Build history of the part. All positions in model axes, mm. A direction names the side the tool comes from. Round coordinates to 2 decimals unless told otherwise and drop trailing zeros. Loops run counter-clockwise (first coordinate to the right, second up) from the corner with the lowest first, then second, coordinate; pieces in that order, holes last. Notation, with made-up numbers: (71, 51.25) - (100, 51.25) arc R30 ccw to (100, 75.25) - close; hole circle Ø1 at (63.25, -33.75). An arc over 180 degrees is marked (long way). Use a Markdown table: item, result.
from build123d import *

# Parameters (mm, degrees)
F0_W          = 59.5
F0_H          = 29.5
F1_DEPTH      = 12.7
F1_DEPTH_BACK = 41.3
F2_R          = 3
F3_DEPTH      = 4.3
F4_R          = 1.5
F5_DEPTH      = 7.8


with BuildPart() as f1:
    # F0 (on Top) → F1 (new body, two sides)
    with BuildSketch(Plane.XY) as f1_sk:
        Rectangle(F0_W, F0_H)
    extrude(amount=F1_DEPTH)
    extrude(f1_sk.sketch, amount=-F1_DEPTH_BACK)

    # F2 (on Top) → F3 (join)
    with BuildSketch(Plane.XY):
        with BuildLine():
            Line((-35.5, -14.75), (35.5, -14.75))
            ThreePointArc((35.5, -14.75), (36.914214, -14.164214), (37.5, -12.75))
            Line((37.5, -12.75), (37.5, 12.75))
            ThreePointArc((37.5, 12.75), (36.914214, 14.164214), (35.5, 14.75))
            Line((35.5, 14.75), (-35.5, 14.75))
            ThreePointArc((-35.5, 14.75), (-36.914214, 14.164214), (-37.5, 12.75))
            Line((-37.5, 12.75), (-37.5, -12.75))
            ThreePointArc((-37.5, -12.75), (-36.914214, -14.164214), (-35.5, -14.75))
        make_face()
        with Locations((-33.476662, -8.75)):
            Circle(F2_R, mode=Mode.SUBTRACT)
        with Locations((34.023338, -8.75)):
            Circle(F2_R, mode=Mode.SUBTRACT)
        with Locations((-33.476662, 8.75)):
            Circle(F2_R, mode=Mode.SUBTRACT)
        with Locations((34.023338, 8.75)):
            Circle(F2_R, mode=Mode.SUBTRACT)
    extrude(amount=F3_DEPTH)

    # F4 (on face) → F5 (join)
    with BuildSketch(Plane.XY.offset(12.7)):
        with Locations((-16.25, 0)):
            Circle(F4_R)
    extrude(amount=F5_DEPTH)


solid = f1.part
Q1. Probe line 1 (Y direction, x = 32, z = 1.5); line 2 (Z direction, x = -13, y = 13); line 3 (X direction, y = -5, z = -12.5). List the from-to ranges inside material, lowest first.
Results found:
| item | result |
|---|---|
| line 1 | y = -14.75 to -10.96, -6.54 to 6.54, 10.96 to 14.75 |
| line 2 | z = -41.3 to 12.7 |
| line 3 | x = -29.75 to 29.75 |
Q2. Pull direction Y, two halves, no side cores. Call faces 5 (the face through (31.026, -8.618, 2.12)), 6 (the face through (0, 0, 12.7)), 7 (the face through (36.93, 14.15, 2.12)), 8 (the face through (-36.474, 8.882, 2.12)): pulls with the +Y half, pulls with the -Y half, needs draft (parallel to the pull), parting line crosses it, or undercut.
Results found:
| item | result |
|---|---|
| face 5 | undercut |
| face 6 | needs draft |
| face 7 | pulls with the +Y half |
| face 8 | undercut |
Q3. Which spindle directions (+Z, -Z, +X, -X, +Y, -Y) get a long thin tool onto all of the face, cutting with end or side? Do faces 1 (the face through (34, 0, 4.3)), 2 (the face through (-29.75, 0, -20)), 3 (the face through (-17.75, 0.07, 16.55)), 4 (the face through (34, 0, 0)). Say none if no direction does.
Results found:
| item | result |
|---|---|
| face 1 | +Z, +X, +Y, -Y |
| face 2 | -Z, -X, +Y, -Y |
| face 3 | +Z |
| face 4 | -Z, +X, +Y, -Y |
Q4. Cut at B-B, the plane x = -16.25. List the corners of the cut face in (y, z).
Results found:
| item | result |
|---|---|
| outline | (-14.75, -41.3) - (14.75, -41.3) - (14.75, 12.7) - (1.5, 12.7) - (1.5, 20.5) - (-1.5, 20.5) - (-1.5, 12.7) - (-14.75, 12.7) - close |
Q5. Drop flat-ended pins along their axis: pin 1 (3 mm diameter, centred on x = 17.5, y = -11, fed in from +Z); pin 2 (4 mm diameter, centred on x = 34.5, y = -7, fed in from +Z); pin 3 (2.5 mm diameter, centred on y = -2, z = 8, fed in from -X); pin 4 (3.5 mm diameter, centred on x = 34.02, y = 8.75, fed in from -Z). Give the stop position or say it passes through.
Results found:
| item | result |
|---|---|
| pin 1 | stops at z = 12.7 |
| pin 2 | stops at z = 4.3 |
| pin 3 | stops at x = -29.75 |
| pin 4 | passes through |
Q6. Cut at D-D, the plane z = -16. List the corners of the cut face in (x, y), plus the area to 3 significant figures.
Results found:
| item | result |
|---|---|
| outline | (-29.75, -14.75) - (29.75, -14.75) - (29.75, 14.75) - (-29.75, 14.75) - close |
| area | 1,760 mm2 |
Q7. Cut at A-A, the plane y = 8.75. List the corners of the cut face in (x, z).
Results found:
| item | result |
|---|---|
| outline | (-37.5, 0) - (-36.48, 0) - (-36.48, 4.3) - (-37.5, 4.3) - close; (-30.48, 0) - (-29.75, 0) - (-29.75, -41.3) - (29.75, -41.3) - (29.75, 0) - (31.02, 0) - (31.02, 4.3) - (29.75, 4.3) - (29.75, 12.7) - (-29.75, 12.7) - (-29.75, 4.3) - (-30.48, 4.3) - close; (37.02, 0) - (37.5, 0) - (37.5, 4.3) - (37.02, 4.3) - close |
Q8. Cut at C-C, the plane y = 0. List the corners of the cut face in (x, z), plus the area to 3 significant figures.
Results found:
| item | result |
|---|---|
| outline | (-37.5, 0) - (-29.75, 0) - (-29.75, -41.3) - (29.75, -41.3) - (29.75, 0) - (37.5, 0) - (37.5, 4.3) - (29.75, 4.3) - (29.75, 12.7) - (-14.75, 12.7) - (-14.75, 20.5) - (-17.75, 20.5) - (-17.75, 12.7) - (-29.75, 12.7) - (-29.75, 4.3) - (-37.5, 4.3) - close |
| area | 3,300 mm2 |
